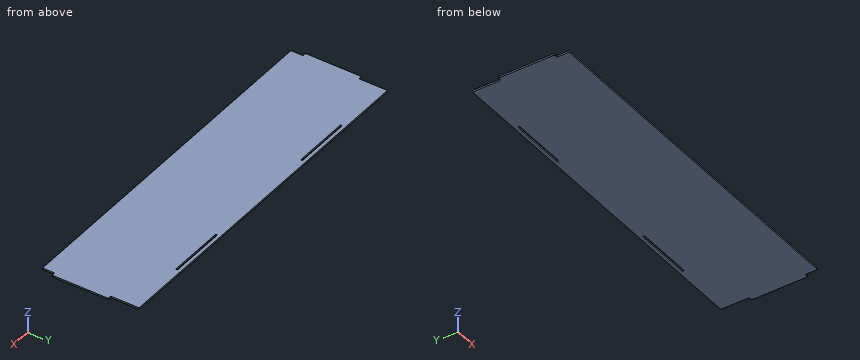
```python
from build123d import *

# Parameters (mm, degrees)
PAD_DEPTH = 1.8542


with BuildPart() as part:
    # Sketch (on Face17 of Binder) → Pad (new body)
    with BuildSketch(Plane.XY.offset(4.0729)):
        with BuildLine():
            Line((-3.0542, 96.721), (-3.0542, 33.379))
            ThreePointArc((-3.0542, 33.379), (-2.702728, 32.530472), (-1.8542, 32.179))
            Line((-1.8542, 32.179), (0, 32.179))
            ThreePointArc((1.2, 30.979), (0.848528, 31.827528), (0, 32.179))
            Line((1.2, 30.979), (1.2, 19.127))
            ThreePointArc((1.2, 19.127), (1.551472, 18.278472), (2.4, 17.927))
            Line((2.4, 17.927), (424.6, 17.927))
            ThreePointArc((424.6, 17.927), (425.448528, 18.278472), (425.8, 19.127))
            Line((425.8, 19.127), (425.8, 30.979))
            ThreePointArc((427, 32.179), (426.151472, 31.827528), (425.8, 30.979))
            Line((427, 32.179), (428.8542, 32.179))
            ThreePointArc((428.8542, 32.179), (429.702728, 32.530472), (430.0542, 33.379))
            Line((430.0542, 33.379), (430.0542, 96.721))
            ThreePointArc((430.0542, 96.721), (429.702728, 97.569528), (428.8542, 97.921))
            Line((428.8542, 97.921), (427, 97.921))
            ThreePointArc((425.8, 99.121), (426.151472, 98.272472), (427, 97.921))
            Line((425.8, 99.121), (425.8, 130.1))
            ThreePointArc((425.8, 130.1), (425.448528, 130.948528), (424.6, 131.3))
            Line((424.6, 131.3), (2.4, 131.3))
            ThreePointArc((2.4, 131.3), (1.551472, 130.948528), (1.2, 130.1))
            Line((1.2, 130.1), (1.2, 99.121))
            ThreePointArc((0, 97.921), (0.848528, 98.272472), (1.2, 99.121))
            Line((0, 97.921), (-1.8542, 97.921))
            ThreePointArc((-1.8542, 97.921), (-2.702728, 97.569528), (-3.0542, 96.721))
        make_face()
        with BuildLine():
            ThreePointArc((73.625, 127.3541), (72.5709, 126.3), (73.625, 125.2459))
            Line((73.625, 125.2459), (139.875, 125.2459))
            ThreePointArc((139.875, 125.2459), (140.9291, 126.3), (139.875, 127.3541))
            Line((73.625, 127.3541), (139.875, 127.3541))
        make_face(mode=Mode.SUBTRACT)
        with BuildLine():
            ThreePointArc((287.125, 127.3541), (286.0709, 126.3), (287.125, 125.2459))
            Line((287.125, 125.2459), (353.375, 125.2459))
            ThreePointArc((353.375, 125.2459), (354.4291, 126.3), (353.375, 127.3541))
            Line((287.125, 127.3541), (353.375, 127.3541))
        make_face(mode=Mode.SUBTRACT)
    extrude(amount=PAD_DEPTH)


solid = part.part
```
Geometry: final body of the model. Coordinates: model frame, mm. Round coordinates to 2 decimals unless told otherwise and drop trailing zeros. Write each loop counter-clockwise with the first axis right and the second up, starting at its lowest first coordinate (ties: lowest second). Pieces come first, ordered by that corner, then holes.
Item 1: Material intervals for L1, parallel to Y at x = 87, z = 4.65; L2, parallel to X at y = 122.5, z = 5.3, sorted ascending.
Item 2: Pin query (flat end, axial travel): P1, Ø0.6, axis at y = 27, z = 4.5, coming from the -X side; P2, Ø0.6, axis at y = 118, z = 5, coming from the +X side. Return the tip coordinate at first contact, or that it passes through.
Item 3: Section query B-B (y = 27). Return loops of the section in (x, z), plus the area to 3 significant figures.
Item 4: Section query A-A (x = 333). Return loops of the section in (y, z).
Completed:
1. L1: y = 17.93 to 125.25, 127.35 to 131.3
1. L2: x = 1.2 to 425.8
2. P1: stops at x = 1.2
2. P2: stops at x = 425.8
3. outline: (1.2, 4.07) - (425.8, 4.07) - (425.8, 5.93) - (1.2, 5.93) - close
3. area: 787 mm2
4. outline: (17.93, 4.07) - (125.25, 4.07) - (125.25, 5.93) - (17.93, 5.93) - close; (127.35, 4.07) - (131.3, 4.07) - (131.3, 5.93) - (127.35, 5.93) - close
